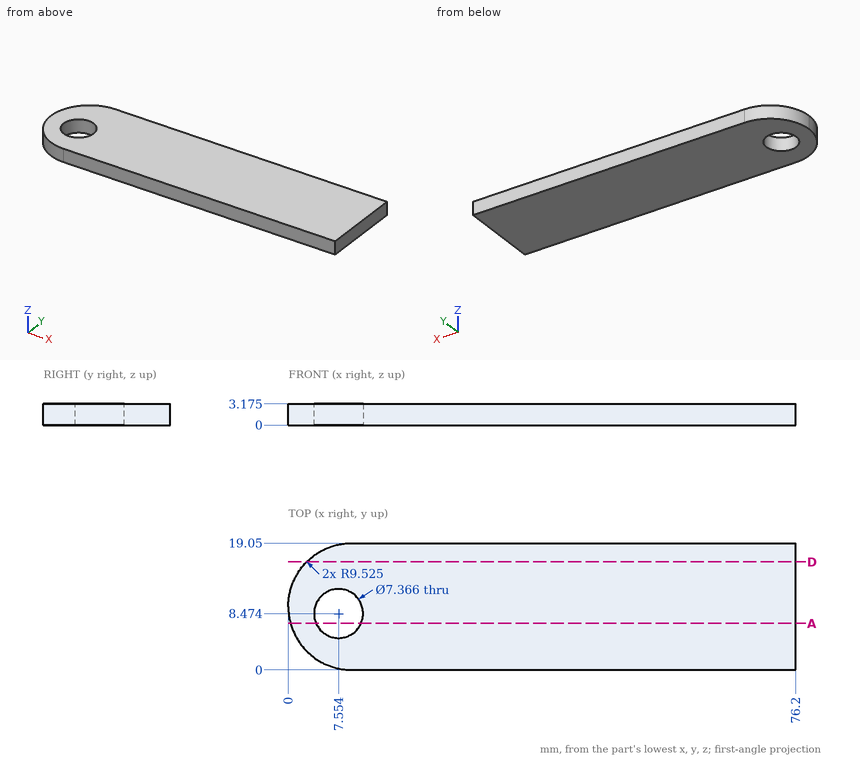
Can you work these out from the drawing? Everything is in mm from the part's minimum corner. Round coordinates to 2 decimals unless told otherwise and drop trailing zeros. Loops run counter-clockwise (first coordinate to the right, second up) from the corner with the lowest first, then second, coordinate; pieces in that order, holes last. Notation, with made-up numbers: (86, 2) - (124, 2) arc R14 cw to (124, 6) - close; hole circle Ø3 at (38.25, 50). An arc over 180 degrees is marked (long way). Answer in a Markdown table with one row per item. Add a question column.
Q1. I want a section at A-A on y = 7. List the corners of the cut face in (x, z) for me (1 decimal).
Q2. I want a section at D-D on y = 16.25. List the corners of the cut face in (x, z) for me (1 decimal).
Q3. I need wall thicknesses on L1, parallel to X at y = 11, z = 1.6 (1 decimal); L2, parallel to Y at x = 5, z = 2.05 (1 decimal); L3, parallel to X at y = 12.25, z = 2.7. Which ranges of each line are inside material? Lowest first, please.
A:
| question | item | result |
|---|---|---|
| 1 | outline | (0.3, 0) - (4.2, 0) - (4.2, 3.2) - (0.3, 3.2) - close; (10.9, 0) - (76.2, 0) - (76.2, 3.2) - (10.9, 3.2) - close |
| 2 | outline | (2.8, 0) - (76.2, 0) - (76.2, 3.2) - (2.8, 3.2) - close |
| 3 | L1 | 0.1 to 4.9, 10.2 to 76.2 |
| 3 | L2 | 1.1 to 5.8, 11.1 to 17.9 |
| 3 | L3 | 0.4 to 76.2 |
